Read the model definition and answer for the solid it produces. Units are mm, in the model's axes. Face numbers are marked on the shaded views. A direction names the side the tool comes from. Give positions to 0.01 mm unless a question says otherwise; leave off trailing zeros. Loops run counter-clockwise (first coordinate to the right, second up) from the corner with the lowest first, then second, coordinate; pieces in that order, holes last.
(1) Which of the six approach directions +Z, -Z, +X, -X, +Y, -Y give full straight-line access (tool end or side, diameter ignored) to the marked faces 1 and 2?
(2) Find section B-B, the plane z = 42.5. Write down the section's boundary in (x, y).
(3) Straight lines are drawn through the part: probe 1 along Z at (x, y) = (61, 10); probe 2 along Y at (x, z) = (-79.35, -44.25); probe 3 along Y at (x, z) = (-48, -31.5). For each, find the intervals that lie inside material, in ascending order.
(4) Find section C-C, the plane x = -64.5. Write down the section's boundary in (y, z), then the cut area to 3 significant figures.
(5) Find section D-D, the plane x = 14. Write down the section's boundary in (y, z).
(6) Each of these flat-tipped pins is pushed along its axis until it touches: P1, Ø1, axis at y = 3, z = 5.5, coming from the -X side; P2, Ø10.5, axis at x = -54.5, z = -9, coming from the +Y side; P3, Ø10, axis at y = 10, z = 8.5, coming from the -X side. Where does it stop, or does it pass through?
(7) Determine the mould class of the marked faces 3 and 4 for opening direction X: pulls with the +X half, pulls with the -X half, needs draft (parallel to the pull), parting line crosses it, or undercut.
```python
from build123d import *

# Parameters (mm, degrees)
ESBO_O1_W                = 163.5
ESBO_O1_H                = 113.5
ESBO_O1_W_2              = 160
ESBO_O1_H_2              = 110
RESSALTO_EXTRUS_O1_DEPTH = 4.8
ESBO_O2_R                = 1
CORTE_EXTRUS_O1_DEPTH    = 20
FILETE1_R                = 2.5
ESBO_O3_W                = 10
ESBO_O3_H                = 5
RESSALTO_EXTRUS_O2_DEPTH = 10
ESBO_O4_W                = 10
ESBO_O4_H                = 50
RESSALTO_EXTRUS_O3_DEPTH = 5
FILETE2_R                = 2.5
FILETE3_R                = 2.5
CORTE_EXTRUS_O2_DEPTH    = 0.5


with BuildPart() as part:
    # Esboço1 → Ressalto-extrusão1 (new body)
    # profile 1 of 2: a face of its own
    with BuildSketch(Plane(origin=(0, 0, 0), x_dir=(1, 0, 0), z_dir=(0, 1, 0))):
        Rectangle(ESBO_O1_W, ESBO_O1_H)
        Rectangle(ESBO_O1_W_2, ESBO_O1_H_2, mode=Mode.SUBTRACT)
    # profile 2 of 2: a face of its own
    with BuildSketch(Plane(origin=(0, 0, 0), x_dir=(1, 0, 0), z_dir=(0, 1, 0))):
        Rectangle(ESBO_O1_W_2, ESBO_O1_H_2)
    extrude(amount=RESSALTO_EXTRUS_O1_DEPTH)

    # Esboço2 → Corte-extrusão1 (cut)
    with BuildSketch(Plane.XY.offset(56.75)):
        with Locations((-79.35, 2.4)):
            Circle(ESBO_O2_R)
        with Locations((79.35, 2.4)):
            Circle(ESBO_O2_R)
    corte_extrus_o1 = extrude(amount=-CORTE_EXTRUS_O1_DEPTH, mode=Mode.SUBTRACT)

    # Espelhar1: Corte-extrusão1 across plane
    add(corte_extrus_o1.mirror(Plane.XY), mode=Mode.SUBTRACT)

    # Filete1
    filete1_edges = [part.edges().sort_by_distance(p)[0] for p in [
        (-81.75, 4.8, 0),
        (81.75, 4.8, 0),
    ]]
    fillet(filete1_edges, radius=FILETE1_R)

    # Esboço3 → Ressalto-extrusão2 (add)
    with BuildSketch(Plane(origin=(0, 4.8, 0), x_dir=(1, 0, 0), z_dir=(0, 1, 0))):
        with Locations((61.75, -22.5)):
            Rectangle(ESBO_O3_W, ESBO_O3_H)
        with Locations((61.75, 22.5)):
            Rectangle(ESBO_O3_W, ESBO_O3_H)
    extrude(amount=RESSALTO_EXTRUS_O2_DEPTH)

    # Esboço4 → Ressalto-extrusão3 (add)
    with BuildSketch(Plane(origin=(0, 14.8, 0), x_dir=(1, 0, 0), z_dir=(0, 1, 0))):
        with Locations((61.75, 0)):
            Rectangle(ESBO_O4_W, ESBO_O4_H)
    extrude(amount=RESSALTO_EXTRUS_O3_DEPTH)

    # Filete2
    filete2_edges = [part.edges().sort_by_distance(p)[0] for p in [
        (61.75, 19.8, -25),
        (61.75, 19.8, 25),
    ]]
    fillet(filete2_edges, radius=FILETE2_R)

    # Filete3
    filete3_edges = [part.edges().sort_by_distance(p)[0] for p in [
        (56.75, 11.05, -25),
        (56.75, 19.067766953, -24.267766953),
        (56.75, 11.05, 25),
        (56.75, 19.067766953, 24.267766953),
        (66.75, 11.05, 25),
        (66.75, 19.067766953, 24.267766953),
        (66.75, 11.05, -25),
        (66.75, 19.067766953, -24.267766953),
        (56.75, 19.8, 0),
        (66.75, 19.8, 0),
        (66.75, 9.8, 20),
        (56.75, 9.8, 20),
        (56.75, 9.8, -20),
        (66.75, 9.8, -20),
    ]]
    fillet(filete3_edges, radius=FILETE3_R - 0.0001)  # a hair under: the kernel refuses the full size

    # Esboço5 → Corte-extrusão2 (cut)
    with BuildSketch(Plane(origin=(0, 4.8, 0), x_dir=(1, 0, 0), z_dir=(0, 1, 0))):
        Polygon((-54.25, 0), (-32.411785944, 60), (-47.411785944, 60), (-69.25, 0), (-47.411785944, -60), (-32.411785944, -60), align=None)
        Polygon((-24.25, 0), (-2.411785944, -60), (-17.411785944, -60), (-39.25, 0), (-17.411785944, 60), (-2.411785944, 60), align=None)
        Polygon((5.75, 0), (27.588214056, -60), (12.588214056, -60), (-9.25, 0), (12.588214056, 60), (27.588214056, 60), align=None)
        Polygon((35.75, 0), (57.588214056, -60), (42.588214056, -60), (20.75, 0), (42.588214056, 60), (57.588214056, 60), align=None)
    extrude(amount=-CORTE_EXTRUS_O2_DEPTH, mode=Mode.SUBTRACT)


solid = part.part
```
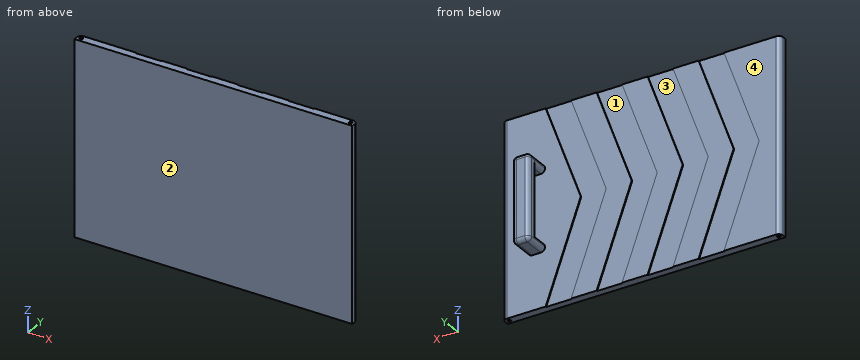
Entries:
1. face 1: +Y
1. face 2: +Z, -Z, +X, -X, -Y
2. outline: (-81.75, 0) - (81.75, 0) - (81.75, 2.3) arc R2.5 ccw to (79.25, 4.8) - (51.22, 4.8) - (51.22, 4.3) - (36.22, 4.3) - (36.22, 4.8) - (21.22, 4.8) - (21.22, 4.3) - (6.22, 4.3) - (6.22, 4.8) - (-8.78, 4.8) - (-8.78, 4.3) - (-23.78, 4.3) - (-23.78, 4.8) - (-38.78, 4.8) - (-38.78, 4.3) - (-53.78, 4.3) - (-53.78, 4.8) - (-79.25, 4.8) arc R2.5 ccw to (-81.75, 2.3) - close; hole circle Ø2 at (-79.35, 2.4); hole circle Ø2 at (79.35, 2.4)
3. probe 1: z = -25 to -20, 20 to 25
3. probe 2: y = 0 to 1.4, 3.4 to 4.8
3. probe 3: y = 0 to 4.3
4. outline: (0, -56.75) - (4.8, -56.75) - (4.8, -13.05) - (4.3, -13.05) - (4.3, 13.05) - (4.8, 13.05) - (4.8, 56.75) - (0, 56.75) - close
4. area: 532 mm2
5. outline: (0, -56.75) - (4.3, -56.75) - (4.3, -22.67) - (4.8, -22.67) - (4.8, 22.67) - (4.3, 22.67) - (4.3, 56.75) - (0, 56.75) - close
6. P1: stops at x = -81.74
6. P2: stops at y = 4.8
6. P3: stops at x = 56.75
7. face 3: undercut
7. face 4: needs draft
